The figure shows three views and two pictorial views of one solid part (mm, origin at its lowest corner). Answer the questions. A direction names the side the tool comes from. Coordinates: 2 decimals unless noted, no trailing zeros. Order: outer loops, then holes, each group sorted by start corner. A loop starts at its lowest first (then second) coordinate and runs counter-clockwise, first axis right, second up. Notation, with made-up numbers: (27, 59) -> (60, 59) arc R22 ccw to (60, 94) -> close; hole circle Ø2 at (-31.5, 24.25). An arc over 180 degrees is marked (long way). Write item = value, one per line. Start each with the question number.
Q1. The part is cut by section B-B, the plane y = 5. Determine the outline of the cut face in (x, z), plus the area to 3 significant figures.
Q2. The part is cut by section D-D, the plane x = 29. Determine the outline of the cut face in (y, z), plus the area to 3 significant figures.
Q3. Which of the six approach directions +Z, -Z, +X, -X, +Y, -Y give full straight-line access (tool end or side, diameter ignored) to the marked faces 4, 5 and 6?
Q4. Straight lines are drawn through the part: L1, parallel to Z at x = 21, y = 0.45; L2, parallel to Z at x = 21, y = 5; L3, parallel to Y at x = 13, z = 13.5. For each, find the intervals that lie inside material, in ascending order. Write a range as from..to.
Q5. The part is cut by section A-A, the plane y = 13. Determine the outline of the cut face in (x, z).
Q6. For a pull along Z with two mould halves and no side action, classify the marked faces 1, 2 and 3 as +Z half, -Z half, draft (parallel to the pull), parting line (faces both ways), or undercut.
Q7. The part is cut by section C-C, the plane x = 36.5. Determine the outline of the cut face in (y, z).
Q8. Flat-ended cylindrical pins translate along their axes: pin 1 (5 mm diameter, centred on x = 21, z = 17, fed in from -Y); pin 2 (2 mm diameter, centred on y = 12, z = 17, fed in from -X); pin 3 (2 mm diameter, centred on x = 5.5, y = 5, fed in from -Z); pin 4 (7 mm diameter, centred on x = 21, z = 17, fed in from +Y). Find the tip coordinate at first contact, or state that the pin passes through.
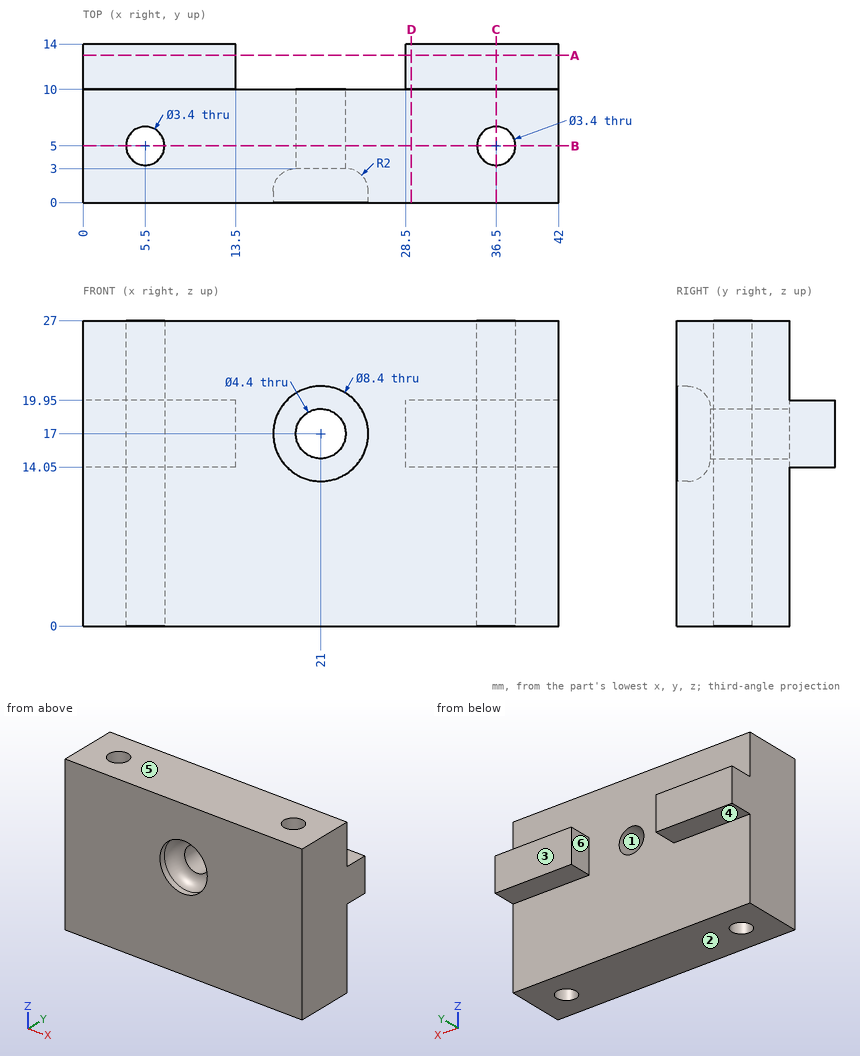
Model answer:
q1.outline = (0, 0) -> (3.8, 0) -> (3.8, 27) -> (0, 27) -> close; (7.2, 0) -> (34.8, 0) -> (34.8, 27) -> (7.2, 27) -> close; (38.2, 0) -> (42, 0) -> (42, 27) -> (38.2, 27) -> close; hole circle Ø4.4 at (21, 17)
q1.area = 935 mm2
q2.outline = (0, 0) -> (10, 0) -> (10, 14.05) -> (14, 14.05) -> (14, 19.95) -> (10, 19.95) -> (10, 27) -> (0, 27) -> close
q2.area = 294 mm2
q3.face_4 = -Z, +X, -X, +Y
q3.face_5 = +Z, +X, -X, +Y, -Y
q3.face_6 = +Z, -Z, +Y
q4.L1 = 0..12.8, 21.2..27
q4.L2 = 0..14.8, 19.2..27
q4.L3 = 0..10
q5.outline = (0, 14.05) -> (13.5, 14.05) -> (13.5, 19.95) -> (0, 19.95) -> close; (28.5, 14.05) -> (42, 14.05) -> (42, 19.95) -> (28.5, 19.95) -> close
q6.face_1 = undercut
q6.face_2 = -Z half
q6.face_3 = draft
q7.outline = (0, 0) -> (3.3, 0) -> (3.3, 27) -> (0, 27) -> close; (6.7, 0) -> (10, 0) -> (10, 14.05) -> (14, 14.05) -> (14, 19.95) -> (10, 19.95) -> (10, 27) -> (6.7, 27) -> close
q8.pin_1 = 2.98
q8.pin_2 = 0
q8.pin_3 = through
q8.pin_4 = 10
